Geometry check sheet. Reference: the model listing, model coordinates, mm. A direction names the side the tool comes from. Coordinates: 2 decimals unless noted, no trailing zeros. Write each loop counter-clockwise with the first axis right and the second up, starting at its lowest first coordinate (ties: lowest second). Pieces come first, ordered by that corner, then holes. Notation, with made-up numbers: (61.5, -9) -> (82.5, -9) arc R23 ccw to (82.5, 4) -> close; hole circle Ø6 at (12.5, 0). An arc over 180 degrees is marked (long way). One line per question, with ' | ' between items.
from build123d import *

# Parameters (mm, degrees)
SKETCH_1_R          = 7
SKETCH_1_R_2        = 2.5
EXTRUDE_1_DEPTH     = 5
SKETCH_2_R          = 6
SKETCH_2_R_2        = 3.5
CUT_EXTRUDE_1_DEPTH = 1
CUT_EXTRUDE_START   = -1
SKETCH_3_R          = 6
SKETCH_3_R_2        = 3.5
CUT_EXTRUDE_2_DEPTH = 1


with BuildPart() as part:
    # 스케치1 → 보스-돌출1 (new body)
    with BuildSketch(Plane(origin=(0, 0, 0), x_dir=(1, 0, 0), z_dir=(0, 1, 0))):
        with Locations(Location((0, 0, 0), (0, 0, 270))):
            Circle(SKETCH_1_R)
        with Locations(Location((0, 0, 0), (0, 0, 270))):
            Circle(SKETCH_1_R_2, mode=Mode.SUBTRACT)
    extrude(amount=EXTRUDE_1_DEPTH)

    # 스케치2 → 컷-돌출1 (cut)
    with BuildSketch(Plane(origin=(0, 5, 0), x_dir=(1, 0, 0), z_dir=(0, 1, 0))):
        with Locations(Location((0, 0, 0), (0, 0, 270))):
            Circle(SKETCH_2_R)
        with Locations(Location((0, 0, 0), (0, 0, 270))):
            Circle(SKETCH_2_R_2, mode=Mode.SUBTRACT)
    extrude(amount=-CUT_EXTRUDE_1_DEPTH, mode=Mode.SUBTRACT)

    # 스케치3 → 컷-돌출2 (cut)
    with BuildSketch(Plane(origin=(0, 0, 0), x_dir=(-1, 0, 0), z_dir=(0, -1, 0)).offset(CUT_EXTRUDE_START)):
        with Locations(Location((0, 0, 0), (0, 0, 270))):
            Circle(SKETCH_3_R)
        with Locations(Location((0, 0, 0), (0, 0, 270))):
            Circle(SKETCH_3_R_2, mode=Mode.SUBTRACT)
    extrude(amount=CUT_EXTRUDE_2_DEPTH, mode=Mode.SUBTRACT)


solid = part.part
1. Cross-section at B-B on x = 0. Record the boundary of the cut face in (y, z), and give its area (3 significant figures).
Worked answers:
outline: (0, -7) -> (5, -7) -> (5, -6) -> (4, -6) -> (4, -3.5) -> (5, -3.5) -> (5, -2.5) -> (0, -2.5) -> (0, -3.5) -> (1, -3.5) -> (1, -6) -> (0, -6) -> close; (0, 2.5) -> (5, 2.5) -> (5, 3.5) -> (4, 3.5) -> (4, 6) -> (5, 6) -> (5, 7) -> (0, 7) -> (0, 6) -> (1, 6) -> (1, 3.5) -> (0, 3.5) -> close | area: 35.0 mm²
2. Cross-section at C-C on y = 0.55. Record the boundary of the cut face in (x, z).
Worked answers:
outline: circle Ø14 at (0, 0); circle Ø7 at (0, 0); hole circle Ø12 at (0, 0); hole circle Ø5 at (0, 0)
3. Cross-section at A-A on z = 0. Record the boundary of the cut face in (x, y).
Worked answers:
outline: (-7, 0) -> (-6, 0) -> (-6, 1) -> (-3.5, 1) -> (-3.5, 0) -> (-2.5, 0) -> (-2.5, 5) -> (-3.5, 5) -> (-3.5, 4) -> (-6, 4) -> (-6, 5) -> (-7, 5) -> close; (2.5, 0) -> (3.5, 0) -> (3.5, 1) -> (6, 1) -> (6, 0) -> (7, 0) -> (7, 5) -> (6, 5) -> (6, 4) -> (3.5, 4) -> (3.5, 5) -> (2.5, 5) -> close
4. Material ranges on line 1 (X direction, y = 0.35, z = 0); line 2 (Z direction, x = -2, y = 4.35), recorded low to high. Write a range as from..to.
Worked answers:
line 1: -7..-6, -3.5..-2.5, 2.5..3.5, 6..7 | line 2: -6.71..-5.66, -2.87..-1.5, 1.5..2.87, 5.66..6.71
5. Cross-section at D-D on x = 4.5. Record the boundary of the cut face in (y, z).
Worked answers:
outline: (0, -5.36) -> (5, -5.36) -> (5, -3.97) -> (4, -3.97) -> (4, 3.97) -> (5, 3.97) -> (5, 5.36) -> (0, 5.36) -> (0, 3.97) -> (1, 3.97) -> (1, -3.97) -> (0, -3.97) -> close
6. Tool access check on faces 1 (the face through (-3.417, 4.507, -0.759)), 2 (the face through (-2, 5, 2)), 3 (the face through (3.417, 0.507, -0.759)). Record the directions out of +Z, -Z, +X, -X, +Y, -Y that give a thin tool (end or side, any length) a straight path to the whole face; none if there is none.
Worked answers:
face 1: +Y | face 2: +Z, -Z, +X, -X, +Y | face 3: -Y
7. Mould release check, pull along X, two halves, no side actions. Record for faces 4 (the face through (-1.802, 0.507, 5.723)), 5 (the face through (2, 5, 6)), 6 (the face through (-6.834, 2.465, -1.517)): released by +X, released by -X, zero draft, split by the parting line, or undercut.
Worked answers:
face 4: undercut | face 5: zero draft | face 6: split by the parting line
8. Go/stop test with flat-tipped pins: P1, Ø1, axis at y = 3.5, z = 5.5, coming from the -X side; P2, Ø3, axis at x = 0, z = 0, coming from the -Y side. Record where each tip stops, or that it passes through.
Worked answers:
P1: x = -4.9 | P2: through
